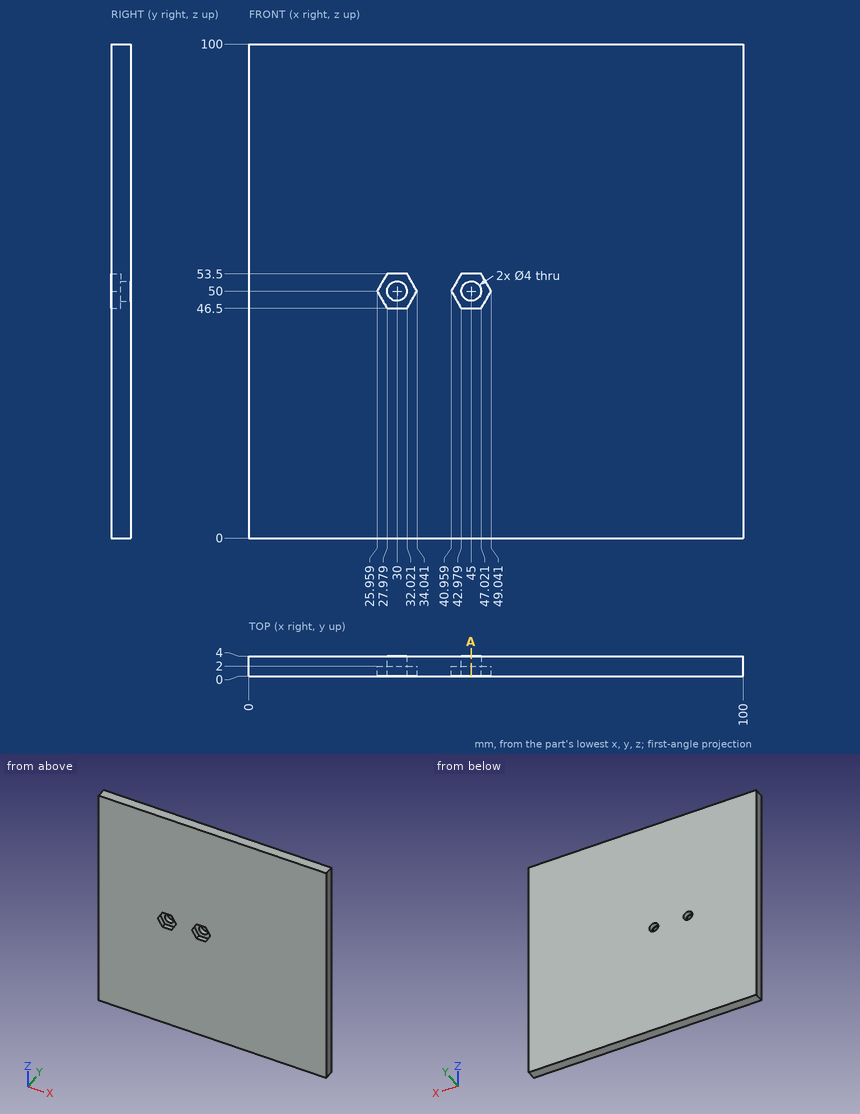
Print and shaded views of the part. All mm, measured from the part's lowest x, y and z. Round coordinates to 2 decimals unless told otherwise and drop trailing zeros. Write each loop counter-clockwise with the first axis right and the second up, starting at its lowest first coordinate (ties: lowest second). Pieces come first, ordered by that corner, then holes.
(1) Drop a flat-ended pin along its axis: P1, Ø3.5, axis at x = 31.5, z = 49.5, coming from the -Y side. Give the stop position or say it passes through.
(2) Probe line 1 along X through (y, z) = (2.9, 50); line 2 along Z through (x, y) = (30, 3.15); line 3 along Z through (x, y) = (48, 0.2) (1 decimal). List the from-to ranges inside material, lowest first.
(3) Slice it at A-A, the plane x = 45. Write the cut outline in (y, z).
From the geometry:
1. P1: stops at y = 2
2. line 1: x = 0 to 28, 32 to 43, 47 to 100
2. line 2: z = 0 to 48, 52 to 100
2. line 3: z = 0 to 48.2, 51.8 to 100
3. outline: (0, 0) - (4, 0) - (4, 48) - (2, 48) - (2, 46.5) - (0, 46.5) - close; (0, 53.5) - (2, 53.5) - (2, 52) - (4, 52) - (4, 100) - (0, 100) - close
